```python
from build123d import *

# Parameters (mm, degrees)
SKETCH1_W             = 7.5000007
SKETCH1_H             = 8
BOSS_EXTRUDE1_DEPTH   = 8
BOSS_EXTRUDE1_2_DEPTH = 8
SKETCH1_W_2           = 7.500000349
SKETCH1_H_2           = 7.999999673
BOSS_EXTRUDE1_3_DEPTH = 8
SKETCH1_W_3           = 7.500000699
SKETCH1_H_3           = 7.999999344
BOSS_EXTRUDE1_4_DEPTH = 8
SKETCH1_W_4           = 7.50000035
SKETCH1_H_4           = 7.999999672
BOSS_EXTRUDE1_5_DEPTH = 8
BOSS_EXTRUDE2_DEPTH   = 2
FILLET1_R             = 1
FILLET2_R             = 1
FILLET3_R             = 1
FILLET4_R             = 1
FILLET5_R             = 1
SHELL8_START          = -2
SHELL8_OUTLINE_W      = 5.5000007
SHELL8_OUTLINE_H      = 6
SHELL8_OUTLINE_W_2    = 5.500000349
SHELL8_OUTLINE_H_2    = 5.999999673
SHELL8_OUTLINE_W_3    = 5.500000699
SHELL8_OUTLINE_H_3    = 5.999999344
SHELL8_OUTLINE_W_4    = 5.50000035
SHELL8_OUTLINE_H_4    = 5.999999672
SHELL8_DEPTH          = 9
SHELL8_2_OUTLINE_W    = 5.50000035
SHELL8_2_OUTLINE_H    = 5.999999672
SHELL8_2_OUTLINE_W_2  = 5.500000699
SHELL8_2_OUTLINE_H_2  = 5.999999344
SHELL8_2_OUTLINE_W_3  = 5.5000007
SHELL8_2_OUTLINE_H_3  = 6
SHELL8_2_OUTLINE_W_4  = 5.500000349
SHELL8_2_OUTLINE_H_4  = 5.999999673
SHELL8_2_DEPTH        = 1


# Read off the part's stored shape, not the designer's step: Shell8
with BuildPart() as part:
    # Sketch1 → Boss-Extrude1 (new body)
    with BuildSketch(Plane.XY):
        with Locations((-28.369785759, -4.064003029)):
            Rectangle(SKETCH1_W, SKETCH1_H)
    extrude(amount=BOSS_EXTRUDE1_DEPTH)



with BuildPart() as body_2:
    # Sketch1 → Boss-Extrude1 2 (new body)
    with BuildSketch(Plane.XY):
        with Locations((-28.369785759, -18.542000511)):
            Rectangle(SKETCH1_W, SKETCH1_H)
    extrude(amount=BOSS_EXTRUDE1_2_DEPTH)


with BuildPart() as body_3:
    # Sketch1 → Boss-Extrude1 3 (new body)
    with BuildSketch(Plane.XY):
        with Locations((-12.748787377, -18.668999085)):
            Rectangle(SKETCH1_W_2, SKETCH1_H_2)
    extrude(amount=BOSS_EXTRUDE1_3_DEPTH)


with BuildPart() as body_4:
    # Sketch1 → Boss-Extrude1 4 (new body)
    with BuildSketch(Plane.XY):
        with Locations((-28.115787957, -33.019997009)):
            Rectangle(SKETCH1_W_3, SKETCH1_H_3)
    extrude(amount=BOSS_EXTRUDE1_4_DEPTH)


with BuildPart() as body_5:
    # Sketch1 → Boss-Extrude1 5 (new body)
    with BuildSketch(Plane.XY):
        with Locations((-43.86378524, -18.795997986)):
            Rectangle(SKETCH1_W_4, SKETCH1_H_4)
    extrude(amount=BOSS_EXTRUDE1_5_DEPTH)


with BuildPart() as part_1:
    add(part.part)

    add(body_2.part)  # Boss-Extrude2 merges body 2

    add(body_3.part)  # Boss-Extrude2 merges body 3

    add(body_4.part)  # Boss-Extrude2 merges body 4

    add(body_5.part)  # Boss-Extrude2 merges body 5
    # Sketch3 → Boss-Extrude2 (add)
    with BuildSketch(Plane(origin=(0, 0, 0), x_dir=(-1, 0, 0), z_dir=(0, 0, -1))):
        Polygon((22.599963615, -12.968328574), (6.599963615, -12.968328574), (6.599963615, -24.568328574), (22.599963615, -24.568328574), (22.599963615, -40.568328574), (34.599963615, -40.568328574), (34.599963615, -24.568328574), (50.599963615, -24.568328574), (50.599963615, -12.968328574), (34.599963615, -12.968328574), (34.599963615, 3.031671426), (22.599963615, 3.031671426), align=None)
    extrude(amount=BOSS_EXTRUDE2_DEPTH)

    # Fillet1
    fillet1_edges = [part_1.edges().sort_by_distance(p)[0] for p in [
        (-31.865788306, -29.019997337, 4),
        (-31.865788306, -37.019996681, 4),
        (-24.365787607, -37.019996681, 4),
        (-24.365787607, -29.019997337, 4),
    ]]
    fillet(fillet1_edges, radius=FILLET1_R)

    # Fillet2
    fillet2_edges = [part_1.edges().sort_by_distance(p)[0] for p in [
        (-32.119786109, -14.542000511, 4),
        (-32.119786109, -22.542000511, 4),
        (-24.619785409, -22.542000511, 4),
        (-24.619785409, -14.542000511, 4),
    ]]
    fillet(fillet2_edges, radius=FILLET2_R)

    # Fillet3
    fillet3_edges = [part_1.edges().sort_by_distance(p)[0] for p in [
        (-47.613785415, -14.79599815, 4),
        (-47.613785415, -22.795997822, 4),
        (-40.113785065, -22.795997822, 4),
        (-40.113785065, -14.79599815, 4),
    ]]
    fillet(fillet3_edges, radius=FILLET3_R)

    # Fillet4
    fillet4_edges = [part_1.edges().sort_by_distance(p)[0] for p in [
        (-32.119786109, -0.064003029, 4),
        (-24.619785409, -0.064003029, 4),
        (-24.619785409, -8.064003029, 4),
        (-32.119786109, -8.064003029, 4),
    ]]
    fillet(fillet4_edges, radius=FILLET4_R)

    # Fillet5
    fillet5_edges = [part_1.edges().sort_by_distance(p)[0] for p in [
        (-16.498787551, -14.668999248, 4),
        (-16.498787551, -22.668998921, 4),
        (-8.998787202, -22.668998921, 4),
        (-8.998787202, -14.668999248, 4),
    ]]
    fillet(fillet5_edges, radius=FILLET5_R)

    # Shell8 outline → Shell8 (cut)
    with BuildSketch(Plane.XY.offset(SHELL8_START)):
        with Locations((-28.369785759, -4.064003029)):
            Rectangle(SHELL8_OUTLINE_W, SHELL8_OUTLINE_H)
        with Locations((-28.369785759, -18.542000511)):
            Rectangle(SHELL8_OUTLINE_W, SHELL8_OUTLINE_H)
        with Locations((-12.748787377, -18.668999085)):
            Rectangle(SHELL8_OUTLINE_W_2, SHELL8_OUTLINE_H_2)
        with Locations((-28.115787957, -33.019997009)):
            Rectangle(SHELL8_OUTLINE_W_3, SHELL8_OUTLINE_H_3)
        with Locations((-43.86378524, -18.795997986)):
            Rectangle(SHELL8_OUTLINE_W_4, SHELL8_OUTLINE_H_4)
    extrude(amount=SHELL8_DEPTH, mode=Mode.SUBTRACT)

    # Shell8 2 outline → Shell8 2 (cut)
    with BuildSketch(Plane.XY.offset(SHELL8_START)):
        Polygon((-23.599963615, -13.968328574), (-23.599963615, 2.031671426), (-33.599963615, 2.031671426), (-33.599963615, -13.968328574), (-49.599963615, -13.968328574), (-49.599963615, -23.568328574), (-33.599963615, -23.568328574), (-33.599963615, -39.568328574), (-23.599963615, -39.568328574), (-23.599963615, -23.568328574), (-7.599963615, -23.568328574), (-7.599963615, -13.968328574), align=None)
        with Locations((-43.86378524, -18.795997986)):
            Rectangle(SHELL8_2_OUTLINE_W, SHELL8_2_OUTLINE_H, mode=Mode.SUBTRACT)
        with Locations((-28.115787957, -33.019997009)):
            Rectangle(SHELL8_2_OUTLINE_W_2, SHELL8_2_OUTLINE_H_2, mode=Mode.SUBTRACT)
        with Locations((-28.369785759, -18.542000511)):
            Rectangle(SHELL8_2_OUTLINE_W_3, SHELL8_2_OUTLINE_H_3, mode=Mode.SUBTRACT)
        with Locations((-12.748787377, -18.668999085)):
            Rectangle(SHELL8_2_OUTLINE_W_4, SHELL8_2_OUTLINE_H_4, mode=Mode.SUBTRACT)
        with Locations((-28.369785759, -4.064003029)):
            Rectangle(SHELL8_2_OUTLINE_W_3, SHELL8_2_OUTLINE_H_3, mode=Mode.SUBTRACT)
    extrude(amount=SHELL8_2_DEPTH, mode=Mode.SUBTRACT)


solid = part_1.part
```
The listing builds one solid part. Answer for the finished solid, in the listing's coordinates (mm). A direction names the side the tool comes from. Coordinates: 2 decimals unless noted, no trailing zeros. Write each loop counter-clockwise with the first axis right and the second up, starting at its lowest first coordinate (ties: lowest second). Pieces come first, ordered by that corner, then holes. Notation, with made-up numbers: M 37,-12 L 84,-12 A16 ccw 84,-3 Z; hole C 1,-4.75 d6. An arc over 180 degrees is marked long. Use a Markdown table: item, result. Add a question column.
1. Straight lines are drawn through the part: line 1 along Y through (x, z) = (-34, -1.5); line 2 along X through (y, z) = (-7, 4.75); line 3 along Y through (x, z) = (-45.5, 5.75). For each, find the intervals that lie inside material, in ascending order. Write a range as [from, to].
2. Section D-D (y = -3) is taken. Give the vertices of the cut face in (x, z), plus the area to 3 significant figures.
3. For a pull along X with two mould halves and no side action, classify faces 1 (the flat face through (-28, -7.064, 3)), 2 (the cylindrical face through (-31.58, -29.32, 4.06)), 3 (the cylindrical face through (-31.835, -22.241, 4.056)), 4 (the flat face through (-13, -19, 8)) as +X half, -X half, draft (parallel to the pull), parting line (faces both ways), or undercut.
4. Given P1, Ø1.8, axis at y = -20, z = 2.5, coming from the +X side; P2, Ø3, axis at y = -26.5, z = -1, coming from the +X side; P3, Ø1, axis at y = -4.5, z = 2.5, coming from the +X side, each flat-ended and moving along its own axis, determine where each tip first touches the part or whether it passes through.
5. Section A-A (y = -11) is taken. Give the vertices of the cut face in (x, z), plus the area to 3 significant figures.
6. Which of the six approach directions +Z, -Z, +X, -X, +Y, -Y give full straight-line access (tool end or side, diameter ignored) to faces 5 (the flat face through (-8.999, -19, 4)), 6 (the flat face through (-28, -22.542, 4)), 7 (the flat face through (-42, -24.568, -1)), 8 (the flat face through (-13, -21.669, 3))?
7. Section C-C (z = 4) is taken. Count the separate pieces of the cut face and the enclosed holes in it, plus the area to 3 significant figures.
8. Section B-B (x = -18.5) is taken. Give the vertices of the cut face in (y, z), plus the area to 3 significant figures.
Data:
| question | item | result |
|---|---|---|
| 1 | line 1 | y = [-40.57, -23.57], [-13.97, 3.03] |
| 1 | line 2 | x = [-32.12, -31.12], [-25.62, -24.62] |
| 1 | line 3 | y = [-22.8, -21.8], [-15.8, -14.8] |
| 2 | outline | M -34.6,-2 L -33.6,-2 L -33.6,-1 L -31.12,-1 L -31.12,7 L -25.62,7 L -25.62,-1 L -23.6,-1 L -23.6,-2 L -22.6,-2 L -22.6,0 L -24.62,0 L -24.62,8 L -32.12,8 L -32.12,0 L -34.6,0 Z |
| 2 | area | 30.0 mm2 |
| 3 | face 1 | undercut |
| 3 | face 2 | -X half |
| 3 | face 3 | undercut |
| 3 | face 4 | draft |
| 4 | P1 | stops at x = -9 |
| 4 | P2 | stops at x = -22.6 |
| 4 | P3 | stops at x = -24.62 |
| 5 | outline | M -34.6,-2 L -33.6,-2 L -33.6,-1 L -23.6,-1 L -23.6,-2 L -22.6,-2 L -22.6,0 L -34.6,0 Z |
| 5 | area | 14.0 mm2 |
| 6 | face 5 | +Z, +X, +Y, -Y |
| 6 | face 6 | +Z |
| 6 | face 7 | +Z, -Z, -X, -Y |
| 6 | face 8 | -Z |
| 7 | separate pieces | 5 |
| 7 | enclosed holes | 5 |
| 7 | area | 131 mm2 |
| 8 | outline | M -24.57,-2 L -23.57,-2 L -23.57,-1 L -13.97,-1 L -13.97,-2 L -12.97,-2 L -12.97,0 L -24.57,0 Z |
| 8 | area | 13.6 mm2 |
